The figure shows three views and two pictorial views of one solid part (mm, origin at its lowest corner). Answer the questions. A direction names the side the tool comes from. Coordinates: 2 decimals unless noted, no trailing zeros. Order: outer loops, then holes, each group sorted by start corner. A loop starts at its lowest first (then second) coordinate and runs counter-clockwise, first axis right, second up.
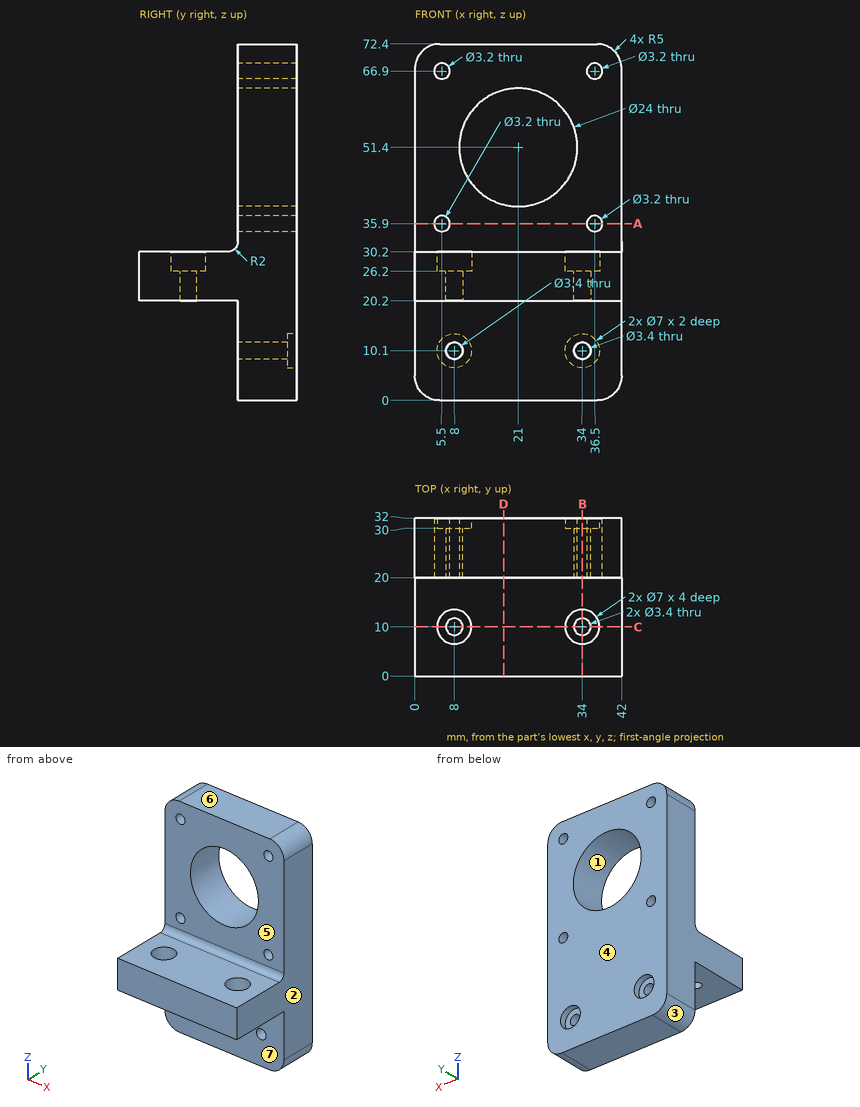
1) Each of these flat-tipped pins is pushed along its axis until it touches: P1, Ø5, axis at x = 36.5, z = 66.9, coming from the -Y side; P2, Ø10, axis at x = 17, z = 47, coming from the +Y side (3 decimals); P3, Ø4, axis at x = 36, y = 3.5, coming from the +Z side; P4, Ø9, axis at x = 34, y = 10, coming from the -Z side. Where does it stop, or does it pass through?
2) The mould has two halves that part along X. Classify the marked faces 1, 2, 3 and 4: released by +X, released by -X, zero draft, split by the parting line, or undercut.
3) For the marked faces 5, 6 and 7, determine the directions among +Z, -Z, +X, -X, +Y, -Y from which every point of the face is accessible in a straight line to the end or side of a thin tool.
4) A cutting plane is placed at D-D, the plane x = 18. Write down the section's boundary in (y, z), plus the area to 3 significant figures.
5) A cutting plane is placed at B-B, the plane x = 34. Write down the section's boundary in (y, z), plus the area to 3 significant figures.
6) Straight lines are drawn through the part: probe 1 along X at (y, z) = (24.5, 51.4); probe 2 along Z at (x, y) = (21, 23); probe 3 along Z at (x, y) = (20.5, 8). For each, find the intervals that lie inside material, in ascending order.
7) A cutting plane is placed at C-C, the plane y = 10. Write down the section's boundary in (x, z).
8) A cutting plane is placed at A-A, the plane z = 35.9. Write down the section's boundary in (x, y).
Working result:
1. P1: stops at y = 20
1. P2: passes through
1. P3: stops at z = 30.2
1. P4: stops at z = 20.2
2. face 1: undercut
2. face 2: released by +X
2. face 3: released by -X
2. face 4: zero draft
3. face 5: +Z, +X, -X, -Y
3. face 6: +Z, +X, -X, +Y, -Y
3. face 7: -Z, +X, -X, -Y
4. outline: (0, 20.2) - (20, 20.2) - (20, 0) - (32, 0) - (32, 39.78) - (20, 39.78) - (20, 32.2) arc R2 cw to (18, 30.2) - (0, 30.2) - close; (20, 63.02) - (32, 63.02) - (32, 72.4) - (20, 72.4) - close
4. area: 791 mm2
5. outline: (0, 20.2) - (8.3, 20.2) - (8.3, 26.2) - (6.5, 26.2) - (6.5, 30.2) - (0, 30.2) - close; (11.7, 20.2) - (20, 20.2) - (20, 11.8) - (30, 11.8) - (30, 13.6) - (32, 13.6) - (32, 72.4) - (20, 72.4) - (20, 32.2) arc R2 cw to (18, 30.2) - (13.5, 30.2) - (13.5, 26.2) - (11.7, 26.2) - close; (20, 0) - (32, 0) - (32, 6.6) - (30, 6.6) - (30, 8.4) - (20, 8.4) - close
5. area: 973 mm2
6. probe 1: x = 0 to 9, 33 to 42
6. probe 2: z = 0 to 39.4, 63.4 to 72.4
6. probe 3: z = 20.2 to 30.2
7. outline: (0, 20.2) - (6.3, 20.2) - (6.3, 26.2) - (4.5, 26.2) - (4.5, 30.2) - (0, 30.2) - close; (9.7, 20.2) - (32.3, 20.2) - (32.3, 26.2) - (30.5, 26.2) - (30.5, 30.2) - (11.5, 30.2) - (11.5, 26.2) - (9.7, 26.2) - close; (35.7, 20.2) - (42, 20.2) - (42, 30.2) - (37.5, 30.2) - (37.5, 26.2) - (35.7, 26.2) - close
8. outline: (0, 20) - (3.9, 20) - (3.9, 32) - (0, 32) - close; (7.1, 20) - (34.9, 20) - (34.9, 32) - (7.1, 32) - close; (38.1, 20) - (42, 20) - (42, 32) - (38.1, 32) - close
